Study the drawing (mm; zero at the part's minimum x, y, z) and answer. Coordinates: 2 decimals unless noted, no trailing zeros. Order: outer loops, then holes, each group sorted by start corner. A loop starts at its lowest first (then second) coordinate and runs counter-clockwise, first axis right, second up. Notation, with made-up numbers: (-2.75, 51.25) -> (20.25, 51.25) arc R16 ccw to (20.25, 60.25) -> close; hole circle Ø10 at (-0.75, -2). An arc over 180 degrees is marked (long way). One line per question, with ' | ' between items.
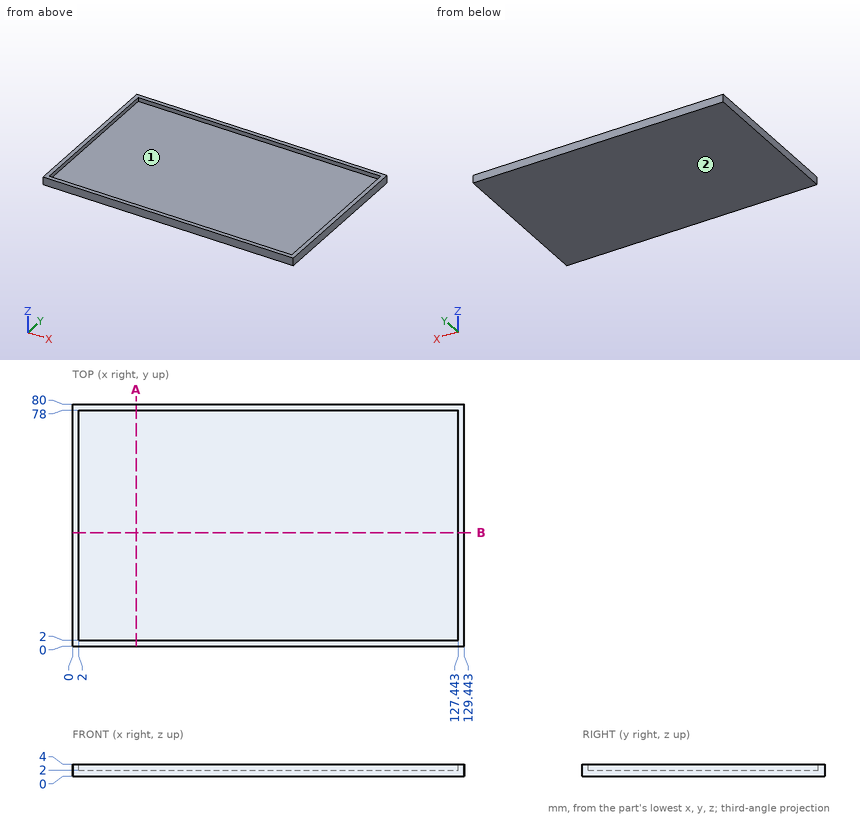
Item 1: Determine the mould class of the marked faces 1 and 2 for opening direction Y: pulls with the +Y half, pulls with the -Y half, needs draft (parallel to the pull), parting line crosses it, or undercut.
Computed values:
face 1: undercut | face 2: needs draft
Item 2: Section B-B, the plane y = 37.5 is taken. Give the vertices of the cut face in (x, z), plus the area to 3 significant figures.
Computed values:
outline: (0, 0) -> (129.44, 0) -> (129.44, 4) -> (127.44, 4) -> (127.44, 2) -> (2, 2) -> (2, 4) -> (0, 4) -> close | area: 267 mm^2
Item 3: Find the intervals of material crossed by L1, parallel to Y at x = 89, z = 3.1; L2, parallel to X at y = 17, z = 3.8; L3, parallel to Z at x = 100, y = 57, in increasing order.
Computed values:
L1: y = 0 to 2, 78 to 80 | L2: x = 0 to 2, 127.44 to 129.44 | L3: z = 0 to 2
Item 4: This flat-tipped pin is pushed along its axis until it touches: pin 1 Ø23 at (x, y) = (37, 43) entering from +Z. Where does it stop, or does it pass through?
Computed values:
pin 1: stops at z = 2
Item 5: Section A-A, the plane x = 21 is taken. Give the vertices of the cut face in (y, z), plus the area to 3 significant figures.
Computed values:
outline: (0, 0) -> (80, 0) -> (80, 4) -> (78, 4) -> (78, 2) -> (2, 2) -> (2, 4) -> (0, 4) -> close | area: 168 mm^2
